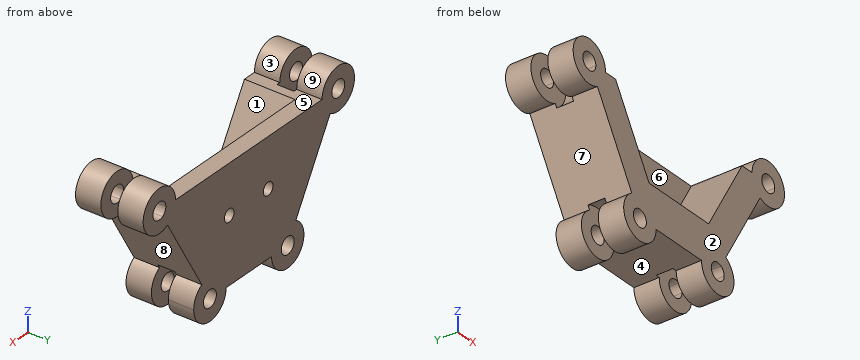
from build123d import *

# Parameters (mm, degrees)
F1_DEPTH = 50.8
F3_DEPTH = 76.2
F4_R     = 38.1
F5_DEPTH = 12.7
F7_R     = 9.525
F8_DEPTH = 50.801


with BuildPart() as f1:
    # F0 (on Front) → F1 (new body, symmetric)
    with BuildSketch(Plane.XZ):
        with BuildLine():
            ThreePointArc((-92.3535701347, -59.3866830272), (-60.6035701347, -59.3866830272), (-44.7285701347, -86.8829895973))
            Line((-44.7285701347, -86.8829895973), (44.1714298653, -86.8829895973))
            ThreePointArc((44.1714298653, -86.8829895973), (60.0464298653, -59.3866830272), (91.7964298653, -59.3866830272))
            Line((91.7964298653, -59.3866830272), (159.0331335179, 57.0707038325))
            ThreePointArc((159.0331335179, 57.0707038325), (147.4118269477, 68.6920104027), (143.1581335179, 84.5670104027))
            Line((143.1581335179, 84.5670104027), (-143.7152737873, 84.5670104027))
            ThreePointArc((-143.7152737873, 84.5670104027), (-147.9689672171, 68.6920104027), (-159.5902737873, 57.0707038325))
            Line((-159.5902737873, 57.0707038325), (-92.3535701347, -59.3866830272))
        make_face()
        with BuildLine():
            ThreePointArc((-143.7152737873, 84.5670104027), (-202.9615803574, 100.4420104027), (-159.5902737873, 57.0707038325))
            Line((-159.5902737873, 57.0707038325), (-169.1152737873, 73.5684877746))
            ThreePointArc((-169.1152737873, 73.5684877746), (-186.4637964153, 90.9170104027), (-162.7652737873, 84.5670104027))
            Line((-162.7652737873, 84.5670104027), (-143.7152737873, 84.5670104027))
        make_face()
        with BuildLine():
            Line((-169.1152737873, 73.5684877746), (-159.5902737873, 57.0707038325))
            ThreePointArc((-159.5902737873, 57.0707038325), (-147.9689672171, 68.6920104027), (-143.7152737873, 84.5670104027))
            Line((-143.7152737873, 84.5670104027), (-162.7652737873, 84.5670104027))
            ThreePointArc((-162.7652737873, 84.5670104027), (-164.4667511592, 78.2170104027), (-169.1152737873, 73.5684877746))
        make_face()
        with BuildLine():
            ThreePointArc((143.1581335179, 84.5670104027), (147.4118269477, 68.6920104027), (159.0331335179, 57.0707038325))
            Line((159.0331335179, 57.0707038325), (168.5581335179, 73.5684877746))
            ThreePointArc((168.5581335179, 73.5684877746), (163.9096108898, 78.2170104027), (162.2081335179, 84.5670104027))
            Line((162.2081335179, 84.5670104027), (143.1581335179, 84.5670104027))
        make_face()
        with BuildLine():
            Line((168.5581335179, 73.5684877746), (159.0331335179, 57.0707038325))
            ThreePointArc((159.0331335179, 57.0707038325), (190.7831335179, 57.0707038325), (206.6581335179, 84.5670104027))
            ThreePointArc((206.6581335179, 84.5670104027), (174.9081335179, 116.3170104027), (143.1581335179, 84.5670104027))
            Line((143.1581335179, 84.5670104027), (162.2081335179, 84.5670104027))
            ThreePointArc((162.2081335179, 84.5670104027), (174.9081335179, 97.2670104027), (187.6081335179, 84.5670104027))
            ThreePointArc((187.6081335179, 84.5670104027), (181.2581335179, 73.5684877746), (168.5581335179, 73.5684877746))
        make_face()
        with BuildLine():
            ThreePointArc((91.7964298653, -59.3866830272), (60.0464298653, -59.3866830272), (44.1714298653, -86.8829895973))
            Line((44.1714298653, -86.8829895973), (63.2214298653, -86.8829895973))
            ThreePointArc((63.2214298653, -86.8829895973), (69.5714298653, -75.8844669693), (82.2714298653, -75.8844669693))
            Line((82.2714298653, -75.8844669693), (91.7964298653, -59.3866830272))
        make_face()
        with BuildLine():
            Line((63.2214298653, -86.8829895973), (44.1714298653, -86.8829895973))
            ThreePointArc((44.1714298653, -86.8829895973), (75.9214298653, -118.6329895973), (107.6714298653, -86.8829895973))
            ThreePointArc((107.6714298653, -86.8829895973), (103.4177364354, -71.0079895973), (91.7964298653, -59.3866830272))
            Line((91.7964298653, -59.3866830272), (82.2714298653, -75.8844669693))
            ThreePointArc((82.2714298653, -75.8844669693), (86.9199524934, -80.5329895973), (88.6214298653, -86.8829895973))
            ThreePointArc((88.6214298653, -86.8829895973), (75.9214298653, -99.5829895973), (63.2214298653, -86.8829895973))
        make_face()
        with BuildLine():
            ThreePointArc((-82.8285701347, -75.8844669693), (-70.1285701347, -75.8844669693), (-63.7785701347, -86.8829895973))
            Line((-63.7785701347, -86.8829895973), (-44.7285701347, -86.8829895973))
            ThreePointArc((-44.7285701347, -86.8829895973), (-60.6035701347, -59.3866830272), (-92.3535701347, -59.3866830272))
            Line((-92.3535701347, -59.3866830272), (-82.8285701347, -75.8844669693))
        make_face()
        with BuildLine():
            Line((-44.7285701347, -86.8829895973), (-63.7785701347, -86.8829895973))
            ThreePointArc((-63.7785701347, -86.8829895973), (-82.8285701347, -97.8815122254), (-82.8285701347, -75.8844669693))
            Line((-82.8285701347, -75.8844669693), (-92.3535701347, -59.3866830272))
            ThreePointArc((-92.3535701347, -59.3866830272), (-92.3535701347, -114.3792961675), (-44.7285701347, -86.8829895973))
        make_face()
    extrude(amount=F1_DEPTH, both=True)

    # F2 (on face) → F3 (cut)
    with BuildSketch(Plane.XZ.offset(50.8)):
        Polygon((123.5816945869, 84.5670104027), (-124.1388348563, 84.5670104027), (-58.6310365333, -28.8958245848), (58.0738962639, -28.8958245848), align=None)
    extrude(amount=-F3_DEPTH, mode=Mode.SUBTRACT)

    # F4 (on Front) → F5 (cut, symmetric)
    with BuildSketch(Plane.XZ):
        with Locations((-176.3127177301, 84.7191157899)):
            Circle(F4_R)
        with Locations((176.0305875596, 85.0320324617)):
            Circle(F4_R)
        with Locations((76.2104084713, -87.0717109253)):
            Circle(F4_R)
        with Locations((-77.118386936, -87.0717109253)):
            Circle(F4_R)
    extrude(amount=F5_DEPTH, both=True, mode=Mode.SUBTRACT)

    # F7 (on face) → F8 (cut, through all)
    with BuildSketch(Plane.XZ):
        with Locations((-38.1, 11.3160433248)):
            Circle(F7_R)
        with Locations((38.1, 11.3160433248)):
            Circle(F7_R)
    extrude(amount=-F8_DEPTH, mode=Mode.SUBTRACT)


solid = f1.part
Geometry: final body of the model. Coordinates: model frame, mm. Face numbers are marked on the shaded views. A direction names the side the tool comes from. Give positions to 0.01 mm unless a question says otherwise; leave off trailing zeros. Loops run counter-clockwise (first coordinate to the right, second up) from the corner with the lowest first, then second, coordinate; pieces in that order, holes last. Notation, with made-up numbers: M 5.5,19.5 L 23.5,19.5 A31 ccw 23.5,57.5 Z; hole C 69.5,43.5 d6. An arc over 180 degrees is marked long. Put each result on its own line as item: value. Start each with the question number.
1) Cut plane C-C (y = 33). Output: boundary loops of the cut face in (x, z) (3 decimals), then the cut area to 3 significant figures.
2) Pull-direction query (Z, two-part tool) for the marked faces 6, 7, 8 and 9; classes: pulls with the +Z half, pulls with the -Z half, needs draft (parallel to the pull), parting line crosses it, or undercut.
3) Access query for the marked faces 1, 2, 3, 4 and 5. Directions: +Z, -Z, +X, -X, +Y, -Y. A direction counts if a zero-diameter tool reaches every point of the face in a straight line with its end or side. Return the directions, or none.
4) Cut plane A-A (y = -38.5). Output: boundary loops of the cut face in (x, z), then the cut area to 3 significant figures.
5) Contact query for flat-ended pins moving along their axis: pin 1 (22 mm diameter, centred on x = -38.1, z = 11.32, fed in from -Y); pin 2 (15 mm diameter, centred on x = -175.47, z = 84.57, fed in from +Y); pin 3 (1 mm diameter, centred on x = -139.5, y = 13.5, fed in from +Z); pin 4 (10 mm diameter, centred on x = -108, y = -26, fed in from +Z). Output: stop coordinate, or through.
6) Ray query, line 1 along Z through (x, y) = (-38.1, 37.75); line 2 along Y through (x, z) = (-163.5, 74.5); line 3 along X through (y, z) = (45, -89). Return the intervals inside material, ascending.
7) Cut plane B-B (z = 16.5). Output: boundary loops of the cut face in (x, y), then the cut area to 3 significant figures.
8) Cut plane D-D (z = 79.5). Give the number of separate pieces and of enclosed holes in the cut face, then the cut area to 3 significant figures.
Verdict:
1. outline: M -159.59,57.071 L -92.354,-59.387 A31.75 ccw long -44.729,-86.883 L 44.171,-86.883 A31.75 ccw long 91.796,-59.387 L 159.033,57.071 A31.75 ccw long 143.158,84.567 L -143.715,84.567 A31.75 ccw long Z; hole C -175.465,84.567 d25.4; hole C -76.479,-86.883 d25.4; hole C -38.1,11.316 d19.05; hole C 38.1,11.316 d19.05; hole C 75.921,-86.883 d25.4; hole C 174.908,84.567 d25.4
1. area: 50,000 mm2
2. face 6: needs draft
2. face 7: undercut
2. face 8: undercut
2. face 9: parting line crosses it
3. face 1: +Z, -Y
3. face 2: +Z, -Z, +X, -X, -Y
3. face 3: +Y, -Y
3. face 4: -Z, +Y, -Y
3. face 5: +Z, +Y, -Y
4. outline: M -159.59,57.07 L -92.35,-59.39 A31.75 ccw long -44.73,-86.88 L 44.17,-86.88 A31.75 ccw long 91.8,-59.39 L 159.03,57.07 A31.75 ccw long 143.16,84.57 L 123.58,84.57 L 58.07,-28.9 L -58.63,-28.9 L -124.14,84.57 L -143.72,84.57 A31.75 ccw long Z; hole C -175.47,84.57 d25.4; hole C -76.48,-86.88 d25.4; hole C 75.92,-86.88 d25.4; hole C 174.91,84.57 d25.4
4. area: 29,900 mm2
5. pin 1: y = 25.4
5. pin 2: through
5. pin 3: z = 84.57
5. pin 4: z = 65.27
6. line 1: -86.88 to 1.79, 20.84 to 84.57
6. line 2: -50.8 to -12.7, 12.7 to 50.8
6. line 3: -108.16 to -89, -63.96 to -44.8, 44.24 to 63.4, 88.44 to 107.6
7. outline: M -136.17,-50.8 L -84.84,-50.8 L -84.84,25.4 L -46.09,25.4 L -46.09,50.8 L -136.17,50.8 Z; M -30.11,25.4 L 30.11,25.4 L 30.11,50.8 L -30.11,50.8 Z; M 46.09,25.4 L 84.28,25.4 L 84.28,-50.8 L 135.61,-50.8 L 135.61,50.8 L 46.09,50.8 Z
7. area: 13,900 mm2
8. separate pieces: 5
8. enclosed holes: 0
8. area: 16,500 mm2
